Design review of the part built by this model. Coordinates are the model's own, in mm. A direction names the side the tool comes from. Round coordinates to 2 decimals unless told otherwise and drop trailing zeros. Order: outer loops, then holes, each group sorted by start corner. A loop starts at its lowest first (then second) coordinate and runs counter-clockwise, first axis right, second up. Notation, with made-up numbers: (58.25, -24) - (75.25, -24) arc R19 ccw to (75.25, 10) - close; hole circle Ø3 at (16, 6). An arc over 180 degrees is marked (long way). Write item = value, one per line.
from build123d import *

# Parameters (mm, degrees)
BOSS_EXTRUDE2_DEPTH = 31.75
SKETCH10_W          = 25.4
SKETCH10_H          = 50.8
CUT_EXTRUDE4_DEPTH  = 32.75
SKETCH11_R          = 2.54
CUT_EXTRUDE5_DEPTH  = 3.175
SKETCH12_R          = 2.54
CUT_EXTRUDE6_DEPTH  = 31.75
SKETCH13_R          = 6.35
CUT_EXTRUDE7_DEPTH  = 3.175


with BuildPart() as part:
    # Sketch8 → Boss-Extrude2 (new body)
    with BuildSketch(Plane.XY):
        Polygon((-15.875, 15.875), (-15.875, -38.1), (15.875, -38.1), (15.875, 38.1), (12.7, 38.1), (12.7, 15.875), align=None)
    extrude(amount=BOSS_EXTRUDE2_DEPTH)

    # Sketch10 → Cut-Extrude4 (cut, through all)
    with BuildSketch(Plane.ZY.offset(15.875)):
        with Locations((15.875, -12.7)):
            Rectangle(SKETCH10_W, SKETCH10_H)
    extrude(amount=-CUT_EXTRUDE4_DEPTH, mode=Mode.SUBTRACT)

    # Sketch11 → Cut-Extrude5 (cut)
    with BuildSketch(Plane(origin=(0, 15.875, 0), x_dir=(1, 0, 0), z_dir=(0, 1, 0))):
        with Locations((-9.525, -15.875)):
            Circle(SKETCH11_R)
        with Locations((3.175, -15.875)):
            Circle(SKETCH11_R)
    extrude(amount=-CUT_EXTRUDE5_DEPTH, mode=Mode.SUBTRACT)

    # Sketch12 → Cut-Extrude6 (cut)
    with BuildSketch(Plane.XY.offset(31.75)):
        with Locations((-3.175, 0)):
            Circle(SKETCH12_R)
        with Locations((-3.175, -12.7)):
            Circle(SKETCH12_R)
        with Locations((-3.175, -25.4)):
            Circle(SKETCH12_R)
    extrude(amount=-CUT_EXTRUDE6_DEPTH, mode=Mode.SUBTRACT)

    # Sketch13 → Cut-Extrude7 (cut)
    with BuildSketch(Plane(origin=(15.875, 0, 0), x_dir=(0, 0, -1), z_dir=(1, 0, 0))):
        with Locations((-15.875, 25.4)):
            Circle(SKETCH13_R)
    extrude(amount=-CUT_EXTRUDE7_DEPTH, mode=Mode.SUBTRACT)


solid = part.part
Item 1: Take a section at C-C, the plane x = -4. Count the separate pieces of the cut face and the enclosed holes in it, and give its area (3 significant figures).
Data:
separate_pieces = 7
enclosed_holes = 0
area = 332 mm2
Item 2: Take a section at B-B, the plane z = 15. State the section outline as (x, y) points (3 decimals).
Data:
outline = (-15.875, 12.7) - (-11.91, 12.7) - (-11.91, 15.875) - (-15.875, 15.875) - close; (-7.14, 12.7) - (0.79, 12.7) - (0.79, 15.875) - (-7.14, 15.875) - close; (5.56, 12.7) - (15.875, 12.7) - (15.875, 19.111) - (12.7, 19.111) - (12.7, 15.875) - (5.56, 15.875) - close; (12.7, 31.689) - (15.875, 31.689) - (15.875, 38.1) - (12.7, 38.1) - close
Item 3: For faces 1 (the face through (12.7, 32, 16)), 2 (the face through (0, -8, 31.75)), 3 (the face through (0, -13, 3.175)), list the 3-axis set-ups (+Z, -Z, +X, -X, +Y, -Y) from which the entire face can be reached by the end or side of a thin tool; tool diameter is ignored.
Data:
face_1 = +Z, -Z, -X, +Y
face_2 = +Z, +X, -X, +Y, -Y
face_3 = +X, -X, -Y
Item 4: For line 1 along Z through (x, y) = (5, 10.5) (3 decimals); line 2 along Y through (x, z) = (3, 21) (3 decimals); line 3 along Y through (x, z) = (13, 8.5), list the stretches that pass through material, from the lowest coordinate up. Write a range as [from, to].
Data:
line_1 = [0, 3.175], [28.575, 31.75]
line_2 = [12.7, 15.875]
line_3 = [12.7, 38.1]
Item 5: The part is to be moulded in two halves that separate along Y. For faces 4 (the face through (0, -38.1, 30)), 5 (the face through (0, -8, 0)), 6 (the face through (-0.75, 0.76, 30.18)), say which applies: +Y half, -Y half, draft (parallel to the pull), parting line (faces both ways), or undercut.
Data:
face_4 = -Y half
face_5 = draft
face_6 = undercut
Item 6: Take a section at D-D, the plane y = 25.4. State the section outline as (x, z) points (3 decimals), and give its area (3 significant figures).
Data:
outline = (12.7, 0) - (15.875, 0) - (15.875, 9.525) - (12.7, 9.525) - close; (12.7, 22.225) - (15.875, 22.225) - (15.875, 31.75) - (12.7, 31.75) - close
area = 60.5 mm2
Item 7: Insertion check: P1, Ø6, axis at x = -1.5, z = 22, coming from the +Y side (3 decimals); P2, Ø1.5, axis at y = 11, z = 10, coming from the +X side. Each pin has a flat end and moves straight along its axis. Give the tip position at first contact, or say it passes through.
Data:
P1 = 15.875
P2 = through
Item 8: Take a section at A-A, the plane y = -12.7. State the section outline as (x, z) points (3 decimals), and give its area (3 significant figures).
Data:
outline = (-15.875, 0) - (-5.715, 0) - (-5.715, 3.175) - (-15.875, 3.175) - close; (-15.875, 28.575) - (-5.715, 28.575) - (-5.715, 31.75) - (-15.875, 31.75) - close; (-0.635, 0) - (15.875, 0) - (15.875, 3.175) - (-0.635, 3.175) - close; (-0.635, 28.575) - (15.875, 28.575) - (15.875, 31.75) - (-0.635, 31.75) - close
area = 169 mm2
